```python
from build123d import *

# Parameters (mm, degrees)
SKETCH2_R                    = 3.282457618
BASE_FLANGE1_DEPTH           = 3.175
EDGE_FLANGE1_STRIP_W         = 19.05
EDGE_FLANGE1_STRIP_H         = 3.175
EDGE_FLANGE1_STRIP_CUT_DEPTH = 37
EDGE_FLANGE1_DEPTH           = 37
SKETCH6_R                    = 3.15
CUT_EXTRUDE1_DEPTH           = 10


# Sheet-metal steps are written as plain solids
with BuildPart() as part:
    # Sketch2 → Base-Flange1 (new body)
    with BuildSketch(Plane(origin=(0, 0, 0), x_dir=(0, 0, -1), z_dir=(1, 0, 0))):
        with BuildLine():
            Line((50.159054546, 37), (50.159054546, 0))
            Line((50.159054546, 0), (67.597909272, 0))
            ThreePointArc((67.597909272, 0), (69.925870777, 0.575003364), (71.718398003, 2.167761907))
            Line((71.718398003, 2.167761907), (95.660507303, 37))
            Line((95.660507303, 37), (50.159054546, 37))
        make_face()
        with Locations((73.009854993, 28.405566411)):
            Circle(SKETCH2_R, mode=Mode.SUBTRACT)
        with Locations((66.344990455, 9.222294526)):
            Circle(SKETCH2_R, mode=Mode.SUBTRACT)
    extrude(amount=-BASE_FLANGE1_DEPTH)

    # Edge-Flange1 strip (across the edge) → Edge-Flange1 strip cut (cut)
    with BuildSketch(Plane(origin=(-3.175, 0, -50.159054546), x_dir=(0, 0, -1), z_dir=(0, 1, 0))):
        with Locations((-3.175, -1.5875)):
            Rectangle(EDGE_FLANGE1_STRIP_W, EDGE_FLANGE1_STRIP_H)
    extrude(amount=EDGE_FLANGE1_STRIP_CUT_DEPTH, mode=Mode.SUBTRACT)

    # Edge-Flange1 section (across the edge) → Edge-Flange1 (add)
    with BuildSketch(Plane(origin=(-3.175, 0, -50.159054546), x_dir=(0, 0, -1), z_dir=(0, 1, 0))):
        with BuildLine():
            Line((0, 3.175), (0, 12.825))
            Line((0, 12.825), (3.175, 12.825))
            Line((3.175, 12.825), (3.175, 3.175))
            ThreePointArc((3.175, 3.175), (4.10493597, 0.92993597), (6.35, 0))
            Line((6.35, 0), (6.35, -3.175))
            ThreePointArc((6.35, -3.175), (1.859871939, -1.315128061), (0, 3.175))
        make_face()
    extrude(amount=EDGE_FLANGE1_DEPTH)

    # Sketch6 → Cut-Extrude1 (cut)
    with BuildSketch(Plane(origin=(0, 0, -53.334054546), x_dir=(-1, 0, 0), z_dir=(0, 0, -1))):
        with Locations((11.175, 28.5)):
            Circle(SKETCH6_R)
        with Locations((11.175, 8.5)):
            Circle(SKETCH6_R)
    extrude(amount=-CUT_EXTRUDE1_DEPTH, mode=Mode.SUBTRACT)


solid = part.part
```
Part model, mm, in its own coordinate system. A direction names the side the tool comes from. Give positions to 0.01 mm unless a question says otherwise; leave off trailing zeros. Order: outer loops, then holes, each group sorted by start corner. A loop starts at its lowest first (then second) coordinate and runs counter-clockwise, first axis right, second up. Notation, with made-up numbers: M -29,60 L -12,60 A20 ccw -12,81 Z; hole C 84.25,73 d11. An arc over 180 degrees is marked long. Use a Markdown table: item, result. Add a question column.
(1) Saw through at A-A, the plane x = -9.25. Give the cut face in (y, z), and give its area (3 significant figures).
(2) Saw through at D-D, the plane x = -1.75. Give the cut face in (y, z) (1 decimal), and give its area (3 significant figures).
(3) Saw through at B-B, the plane z = -66.5. Give the cut face in (x, y) (1 decimal).
(4) Mould opens along Y. For faces 1 (the face through (-1.565, 7.225, -63.74)), 2 (the face through (-11, 18, -53.334)), 3 (the face through (-1.57, 19.34, -83.52)) say: +Y half, -Y half, draft (parallel to the pull), parting line (faces both ways), or undercut.
(5) Saw through at C-C, the plane y = 8.5. Give the cut face in (x, z) (3 decimals).
(6) Drop flat-ended pins along their axis: P1, Ø12, axis at y = 11, z = -60, coming from the -X side; P2, Ø5, axis at x = -9.5, y = 18.5, coming from the -Z side; P3, Ø10, axis at y = 23, z = -70, coming from the -X side (3 decimals). Give the stop position or say it passes through.
(7) Probe line 1 along X through (y, z) = (35, -68) (3 decimals); line 2 along Z through (x, y) = (-13.5, 16); line 3 along X through (y, z) = (8, -51). List the from-to ranges inside material, lowest first. Write a range as [from, to].
(8) 3-axis set-ups, long thin cutter, end or side, ignore diameter. For faces 4 (the face through (-3.175, 23, -71)), 5 (the face through (0, 23, -71)): which of +Z, -Z, +X, -X, +Y, -Y reach the whole face in a straight line?
Answer key:
| question | item | result |
|---|---|---|
| 1 | outline | M 0,-53.33 L 6.01,-53.33 L 6.01,-50.16 L 0,-50.16 Z; M 10.99,-53.33 L 26.01,-53.33 L 26.01,-50.16 L 10.99,-50.16 Z; M 30.99,-53.33 L 37,-53.33 L 37,-50.16 L 30.99,-50.16 Z |
| 1 | area | 85.8 mm^2 |
| 2 | outline | M 0,-67.6 A5 ccw 2.2,-71.7 L 37,-95.7 L 37,-52.1 L 0,-52.1 Z; hole C 9.2,-66.3 d6.6; hole C 28.4,-73 d6.6 |
| 2 | area | 1,070 mm^2 |
| 3 | outline | M -3.2,0 L 0,0 L 0,5.9 L -3.2,5.9 Z; M -3.2,12.5 L 0,12.5 L 0,37 L -3.2,37 Z |
| 4 | face 1 | undercut |
| 4 | face 2 | draft |
| 4 | face 3 | -Y half |
| 5 | outline | M -16,-53.334 L -14.325,-53.334 L -14.325,-50.159 L -16,-50.159 Z; M -8.025,-53.334 L -6.35,-53.334 A3.175 cw -3.175,-56.509 L -3.175,-63.143 L 0,-63.143 L 0,-56.509 A6.35 ccw -6.35,-50.159 L -8.025,-50.159 Z; M -3.175,-76.071 L 0,-76.071 L 0,-69.547 L -3.175,-69.547 Z |
| 6 | P1 | x = -4.4 |
| 6 | P2 | z = -53.33 |
| 6 | P3 | x = -3.175 |
| 7 | line 1 | [-3.175, 0] |
| 7 | line 2 | [-53.33, -50.16] |
| 7 | line 3 | [-16, -14.29], [-8.06, -3.19] |
| 8 | face 4 | -Z, -X, +Y, -Y |
| 8 | face 5 | +Z, -Z, +X, +Y, -Y |
